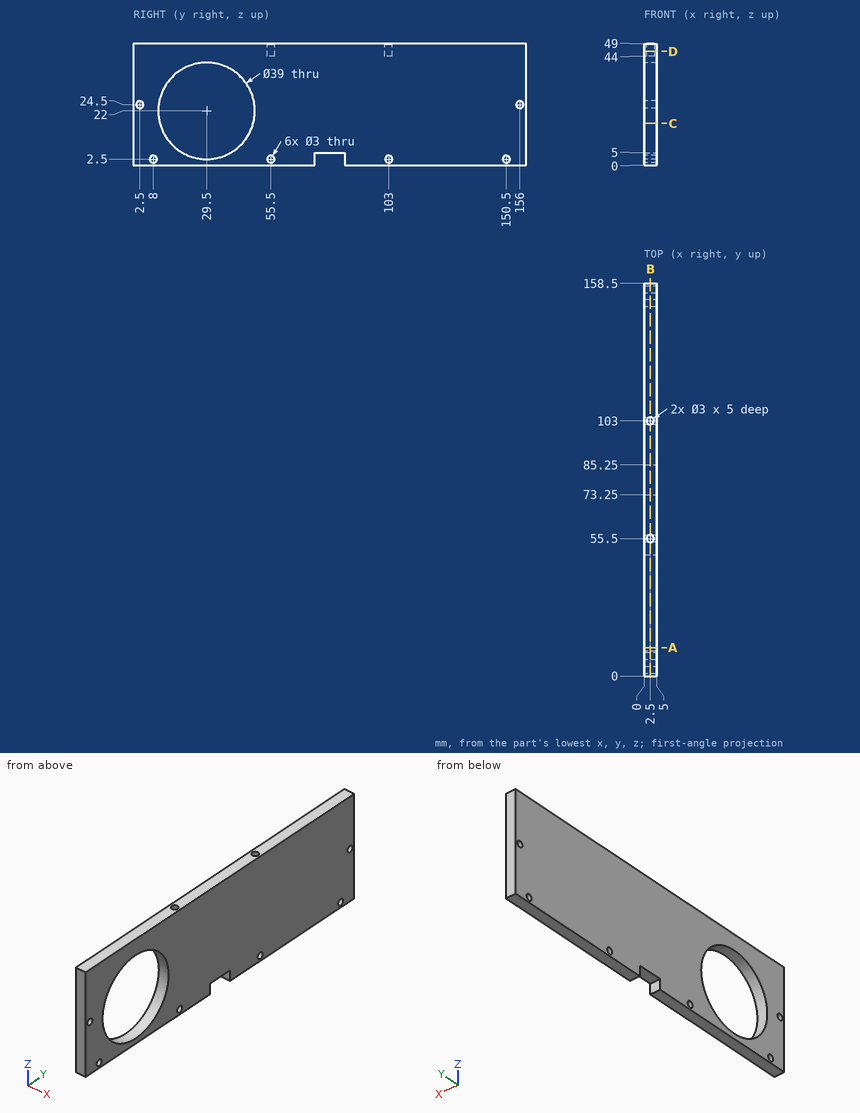
Can you work these out from the drawing? Everything is in mm from the part's minimum corner. Round coordinates to 2 decimals unless told otherwise and drop trailing zeros. Order: outer loops, then holes, each group sorted by start corner. A loop starts at its lowest first (then second) coordinate and runs counter-clockwise, first axis right, second up. Notation, with made-up numbers: M 53,61 L 110,61 A12 ccw 110,67 Z; hole C 54,-5.75 d7. An arc over 180 degrees is marked long. Answer as CSV lines item,"result".
Item 1: Imagine slicing it at A-A on y = 11.5. List the corners of the cut face in (x, z) for me, and give its area (3 significant figures).
From the geometry:
outline,"M 0,0 L 5,0 L 5,14.5 L 0,14.5 Z; M 0,29.5 L 5,29.5 L 5,49 L 0,49 Z"
area,"170 mm2"
Item 2: Imagine slicing it at D-D on z = 46. List the corners of the cut face in (x, y) for me, and give its area (3 significant figures).
From the geometry:
outline,"M 0,0 L 5,0 L 5,158.5 L 0,158.5 Z; hole C 2.5,55.5 d3; hole C 2.5,103 d3"
area,"778 mm2"
Item 3: For pin 1 (2.5 mm diameter, centred on x = 2.5, y = 55.5, fed in from -Z); pin 2 (1.5 mm diameter, centred on x = 3.5, y = 82, fed in from -Z); pin 3 (1.8 mm diameter, centred on y = 156, z = 24.5, fed in from -X), each with a flat end and sliding along its axis, tell me the tip position at first contact or that it passes through.
From the geometry:
pin 1,"z = 0"
pin 2,"z = 5"
pin 3,"through"
Item 4: Imagine slicing it at C-C on z = 17. List the corners of the cut face in (x, y) for me, and give its area (3 significant figures).
From the geometry:
outline,"M 0,0 L 5,0 L 5,10.65 L 0,10.65 Z; M 0,48.35 L 5,48.35 L 5,158.5 L 0,158.5 Z"
area,"604 mm2"
Item 5: Imagine slicing it at B-B on x = 2.5. List the corners of the cut face in (y, z) for me.
From the geometry:
outline,"M 0,0 L 73.25,0 L 73.25,5 L 85.25,5 L 85.25,0 L 158.5,0 L 158.5,49 L 104.5,49 L 104.5,44 L 101.5,44 L 101.5,49 L 57,49 L 57,44 L 54,44 L 54,49 L 0,49 Z; hole C 2.5,24.5 d3; hole C 8,2.5 d3; hole C 29.5,22 d39; hole C 55.5,2.5 d3; hole C 103,2.5 d3; hole C 150.5,2.5 d3; hole C 156,24.5 d3"
Item 6: Please list where these lines run through material, in increasing order: L1, parallel to X at y = 103, z = 45.65; L2, parallel to Z at x = 2.8, y = 103; L3, parallel to Z at x = 3.4, y = 2.5. Write a range as [from, to].
From the geometry:
L1,"[0, 1], [4, 5]"
L2,"[0, 1], [4, 44]"
L3,"[0, 23], [26, 49]"
